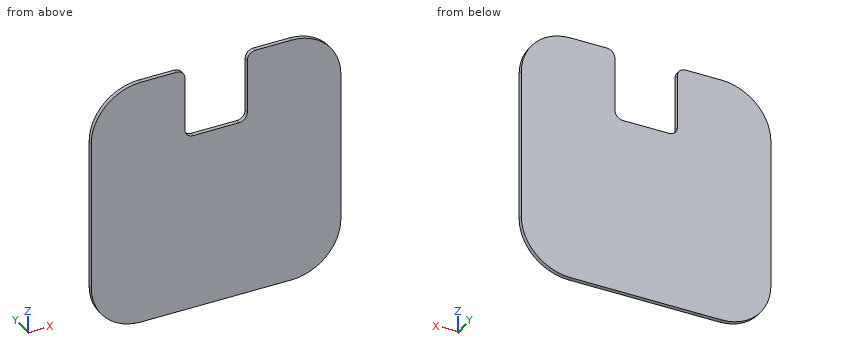
from build123d import *

# Parameters (mm, degrees)
BOSS_EXTRUDE1_DEPTH = 1
SKETCH3_W           = 15
SKETCH3_H           = 17
CUT_EXTRUDE1_DEPTH  = 1
FILLET1_R           = 2


with BuildPart() as part:
    # Sketch2 → Boss-Extrude1 (new body)
    with BuildSketch(Plane(origin=(0, 0, 0), x_dir=(1, 0, 0), z_dir=(0, 1, 0))):
        with BuildLine():
            Line((-18.106601718, -30), (18.106601718, -30))
            ThreePointArc((18.106601718, -30), (26.516504294, -26.516504294), (30, -18.106601718))
            Line((30, -18.106601718), (30, 18.106601718))
            ThreePointArc((30, 18.106601718), (26.516504294, 26.516504294), (18.106601718, 30))
            Line((18.106601718, 30), (-18.106601718, 30))
            ThreePointArc((-18.106601718, 30), (-26.516504294, 26.516504294), (-30, 18.106601718))
            Line((-30, 18.106601718), (-30, -18.106601718))
            ThreePointArc((-30, -18.106601718), (-26.516504294, -26.516504294), (-18.106601718, -30))
        make_face()
    extrude(amount=BOSS_EXTRUDE1_DEPTH)

    # Sketch3 → Cut-Extrude1 (cut)
    with BuildSketch(Plane(origin=(0, 0, 0), x_dir=(1, 0, 0), z_dir=(0, 1, 0))):
        with Locations((0, -21.5)):
            Rectangle(SKETCH3_W, SKETCH3_H)
    extrude(amount=CUT_EXTRUDE1_DEPTH, mode=Mode.SUBTRACT)

    # Fillet1
    fillet1_edges = [part.edges().sort_by_distance(p)[0] for p in [
        (-7.5, 0.5, 13),
        (-7.5, 0.5, 30),
        (7.5, 0.5, 30),
        (7.5, 0.5, 13),
    ]]
    fillet(fillet1_edges, radius=FILLET1_R)


solid = part.part
The listing builds one solid part. Answer for the finished solid, in the listing's coordinates (mm). Give positions to 0.01 mm unless a question says otherwise; leave off trailing zeros. Order: outer loops, then holes, each group sorted by start corner. A loop starts at its lowest first (then second) coordinate and runs counter-clockwise, first axis right, second up. Notation, with made-up numbers: (68, 31.5) -> (76, 31.5) arc R24 ccw to (76, 56.5) -> close; hole circle Ø9 at (71, 89). An arc over 180 degrees is marked (long way). Put each result on its own line as item: value.
Item 1: A cutting plane is placed at A-A on z = 21.5. Give the vertices of the cut face in (x, y).
Established:
outline: (-29.51, 0) -> (-7.5, 0) -> (-7.5, 1) -> (-29.51, 1) -> close; (7.5, 0) -> (29.51, 0) -> (29.51, 1) -> (7.5, 1) -> close
Item 2: A cutting plane is placed at D-D on z = -23.5. Give the vertices of the cut face in (x, y), plus the area to 3 significant figures.
Established:
outline: (-28.71, 0) -> (28.71, 0) -> (28.71, 1) -> (-28.71, 1) -> close
area: 57.4 mm^2
Item 3: A cutting plane is placed at B-B on y = 0.6. Give the vertices of the cut face in (x, z), plus the area to 3 significant figures.
Established:
outline: (-30, -18.11) arc R11.89 ccw to (-18.11, -30) -> (18.11, -30) arc R11.89 ccw to (30, -18.11) -> (30, 18.11) arc R11.89 ccw to (18.11, 30) -> (9.5, 30) arc R2 ccw to (7.5, 28) -> (7.5, 15) arc R2 cw to (5.5, 13) -> (-5.5, 13) arc R2 cw to (-7.5, 15) -> (-7.5, 28) arc R2 ccw to (-9.5, 30) -> (-18.11, 30) arc R11.89 ccw to (-30, 18.11) -> close
area: 3,220 mm^2
Item 4: Straight lines are drawn through the part: line 1 (Z direction, x = -0.5, y = 0.15); line 2 (Z direction, x = 9, y = 0.65); line 3 (X direction, y = 0.65, z = 13.5). For each, find the intervals that lie inside material, in ascending order.
Established:
line 1: z = -30 to 13
line 2: z = -30 to 29.94
line 3: x = -30 to -6.82, 6.82 to 30
Item 5: A cutting plane is placed at C-C on x = -2. Give the vertices of the cut face in (y, z), plus the area to 3 significant figures.
Established:
outline: (0, -30) -> (1, -30) -> (1, 13) -> (0, 13) -> close
area: 43.0 mm^2
